The listing builds one solid part. Answer for the finished solid, in the listing's coordinates (mm). A direction names the side the tool comes from. Round coordinates to 2 decimals unless told otherwise and drop trailing zeros. Write each loop counter-clockwise with the first axis right and the second up, starting at its lowest first coordinate (ties: lowest second). Pieces come first, ordered by that corner, then holes.
Item 1: Find section D-D on z = 7.25. Give the vertices of the cut face in (x, y), then the cut area to 3 significant figures.
Item 2: Each of these flat-tipped pins is pushed along its axis until it touches: pin 1 (6 mm diameter, centred on x = 18.5, y = 9.5, fed in from -Z); pin 2 (2 mm diameter, centred on y = 45.5, z = 5, fed in from +X); pin 3 (4 mm diameter, centred on x = 12.5, z = -5, fed in from +Y); pin 4 (6 mm diameter, centred on x = 2, y = 23, fed in from -Z). Where does it stop, or does it pass through?
Item 3: Find section A-A on y = 45. Give the vertices of the cut face in (x, z).
Item 4: Find section B-B on x = 5.75. Give the vertices of the cut face in (y, z).
Item 5: A tool of negligible diameter and unlimited length cuts with its end or side. For faces 5 (the face through (5, 29, 10.958)), 6 (the face through (9.4, 25.45, 9.44)), 7 (the face through (11, 35, 7.958)), from which of +Z, -Z, +X, -X, +Y, -Y can it reach the whole face along a straight path? Write none if from no direction.
Item 6: For a pull along X with two mould halves and no side action, classify faces 1 (the face through (21.078, 20, 9)), 2 (the face through (19.37, 7.93, 4.41)), 3 (the face through (6.328, 40, 9)), 4 (the face through (8, 3, 1)) as +X half, -X half, draft (parallel to the pull), parting line (faces both ways), or undercut.
Item 7: Find section C-C on x = 18.75. Give the vertices of the cut face in (y, z).
Item 8: Find the intervals of material crossed by probe 1 along X at (y, z) = (31.5, 8.75); probe 2 along Z at (x, y) = (3, 18); probe 3 along Y at (x, z) = (12, 9.25), in increasing order.
```python
from build123d import *

# Parameters (mm, degrees)
ESBO_O1_W                = 26
ESBO_O1_H                = 20
RESSALTO_EXTRUS_O1_DEPTH = 3
ESBO_O2_W                = 26
ESBO_O2_H                = 3
RESSALTO_EXTRUS_O2_DEPTH = 55
ESBO_O3_W                = 3
ESBO_O3_H                = 7
RESSALTO_EXTRUS_O3_DEPTH = 10
CORTE_EXTRUS_O1_DEPTH    = 65.498700042
CORTE_EXTRUS_O2_REACH    = 66.01
ESBO_O6_W                = 20
ESBO_O6_H                = 10
FILETE1_R                = 3
CORTE_EXTRUS_O3_REACH    = 66.871
ESBO_O7_W                = 1.75
ESBO_O7_H                = 30
FILETE2_R                = 1.5


with BuildPart() as part:
    # Esboço1 → Ressalto-extrusão1 (new body)
    with BuildSketch(Plane(origin=(0, 0, 0), x_dir=(1, 0, 0), z_dir=(0, 1, 0))):
        with Locations((8.077993659, -0.958207295)):
            Rectangle(ESBO_O1_W, ESBO_O1_H)
    extrude(amount=RESSALTO_EXTRUS_O1_DEPTH)

    # Esboço2 → Ressalto-extrusão2 (add)
    with BuildSketch(Plane(origin=(0, 3, 0), x_dir=(1, 0, 0), z_dir=(0, 1, 0))):
        with Locations((8.077993659, -9.458207295)):
            Rectangle(ESBO_O2_W, ESBO_O2_H)
    extrude(amount=RESSALTO_EXTRUS_O2_DEPTH)

    # Esboço3 → Ressalto-extrusão3 (add)
    with BuildSketch(Plane(origin=(0, 3, 0), x_dir=(1, 0, 0), z_dir=(0, 1, 0))):
        with Locations((19.577993659, -4.458207295)):
            Rectangle(ESBO_O3_W, ESBO_O3_H)
        with Locations((-3.422006341, -4.458207295)):
            Rectangle(ESBO_O3_W, ESBO_O3_H)
    extrude(amount=RESSALTO_EXTRUS_O3_DEPTH)

    # Esboço4 → Corte-extrusão1 (cut, through all)
    with BuildSketch(Plane.ZY.offset(4.922006341)):
        Polygon((0.958207295, 3), (7.958207295, 13), (0.958207295, 13), align=None)
    extrude(amount=-CORTE_EXTRUS_O1_DEPTH, mode=Mode.SUBTRACT)

    # Esboço6 → Corte-extrusão2 (cut, up to next)
    with BuildSketch(Plane(origin=(0, 0, 7.958207295), x_dir=(-1, 0, 0), z_dir=(0, 0, -1)), mode=Mode.PRIVATE) as corte_extrus_o2_sk1:
        with Locations((-8.077993659, 8)):
            Rectangle(ESBO_O6_W, ESBO_O6_H)
    corte_extrus_o2_tool1 = extrude(corte_extrus_o2_sk1.sketch, amount=-CORTE_EXTRUS_O2_REACH, mode=Mode.PRIVATE) & part.part
    add(corte_extrus_o2_tool1.solids().sort_by_distance((8.077994, 8, 7.958207))[0], mode=Mode.SUBTRACT)

    # Filete1
    filete1_edges = [part.edges().sort_by_distance(p)[0] for p in [
        (18.077993659, 13, 9.458207295),
        (-1.922006341, 13, 9.458207295),
    ]]
    fillet(filete1_edges, radius=FILETE1_R)

    # Esboço7 → Corte-extrusão3 (cut, up to next)
    with BuildSketch(Plane.XY.offset(10.958207295), mode=Mode.PRIVATE) as corte_extrus_o3_sk1:
        with Locations((7.202993659, 40)):
            Rectangle(ESBO_O7_W, ESBO_O7_H)
    corte_extrus_o3_tool1 = extrude(corte_extrus_o3_sk1.sketch, amount=-CORTE_EXTRUS_O3_REACH, mode=Mode.PRIVATE) & part.part
    # Esboço7 → Corte-extrusão3 (cut, up to next)
    with BuildSketch(Plane.XY.offset(10.958207295), mode=Mode.PRIVATE) as corte_extrus_o3_sk2:
        with Locations((8.952993659, 40)):
            Rectangle(ESBO_O7_W, ESBO_O7_H)
    corte_extrus_o3_tool2 = extrude(corte_extrus_o3_sk2.sketch, amount=-CORTE_EXTRUS_O3_REACH, mode=Mode.PRIVATE) & part.part
    add(corte_extrus_o3_tool1.solids().sort_by_distance((7.202994, 40, 10.958207))[0], mode=Mode.SUBTRACT)
    add(corte_extrus_o3_tool2.solids().sort_by_distance((8.952994, 40, 10.958207))[0], mode=Mode.SUBTRACT)

    # Filete2
    filete2_edges = [part.edges().sort_by_distance(p)[0] for p in [
        (9.827993659, 25, 9.458207295),
        (6.327993659, 25, 9.458207295),
        (6.327993659, 55, 9.458207295),
        (9.827993659, 55, 9.458207295),
    ]]
    fillet(filete2_edges, radius=FILETE2_R)


solid = part.part
```
Check values:
1. outline: (-4.92, 0) - (21.08, 0) - (21.08, 11.99) - (17.32, 11.99) arc R3 cw to (18.08, 10) - (18.08, 3) - (-1.92, 3) - (-1.92, 10) arc R3 cw to (-1.17, 11.99) - (-4.92, 11.99) - close
1. area: 133 mm2
2. pin 1: stops at z = 3.41
2. pin 2: passes through
2. pin 3: stops at y = 3
2. pin 4: stops at z = 7.96
3. outline: (-4.92, 7.96) - (6.33, 7.96) - (6.33, 10.96) - (-4.92, 10.96) - close; (9.83, 7.96) - (21.08, 7.96) - (21.08, 10.96) - (9.83, 10.96) - close
4. outline: (0, -9.04) - (3, -9.04) - (3, 10.96) - (0, 10.96) - close; (13, 7.96) - (58, 7.96) - (58, 10.96) - (13, 10.96) - close
5. face 5: +Z, +X, -X, +Y, -Y
5. face 6: +Z, -Z
5. face 7: -Z, +X, -X, +Y
6. face 1: +X half
6. face 2: draft
6. face 3: undercut
6. face 4: undercut
7. outline: (0, -9.04) - (3, -9.04) - (3, 0.96) - (13, 7.96) - (58, 7.96) - (58, 10.96) - (0, 10.96) - close
8. probe 1: x = -4.92 to 6.33, 9.83 to 21.08
8. probe 2: z = 7.96 to 10.96
8. probe 3: y = 0 to 3, 13 to 58
